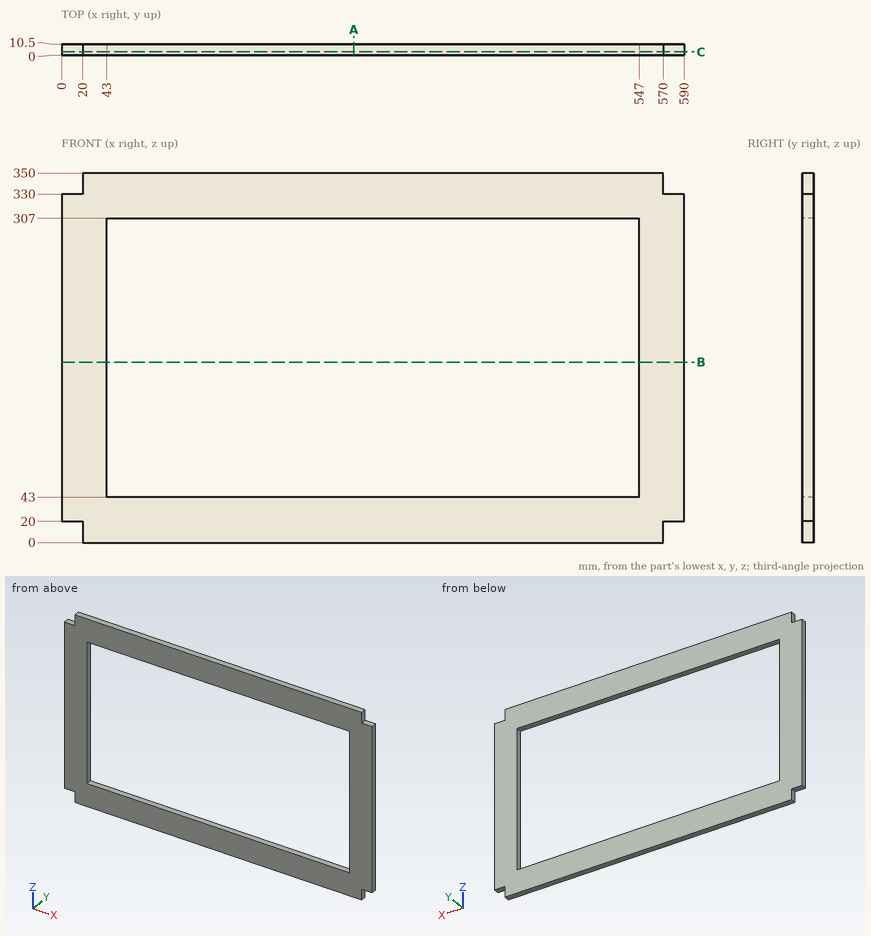
Can you work these out from the drawing? Everything is in mm from the part's minimum corner. Give positions to 0.01 mm unless a question says otherwise; leave off trailing zeros. Loops run counter-clockwise (first coordinate to the right, second up) from the corner with the lowest first, then second, coordinate; pieces in that order, holes last. Notation, with made-up numbers: (32.5, 36) -> (66.5, 36) arc R21 ccw to (66.5, 69) -> close; hole circle Ø10 at (12, 36). An arc over 180 degrees is marked (long way). Write item = value, one per line.
1) I need wall thicknesses on L1, parallel to X at y = 8, z = 279.5; L2, parallel to Z at x = 325.5, y = 8.75. Which ranges of each line are inside material? Lowest first, please. Write a range as from..to.
Check result:
L1 = 0..43, 547..590
L2 = 0..43, 307..350
2) Suppose I cut it at B-B on z = 171. Write out the boundary of the cut face in (x, y), then the cut area to 3 significant figures.
Check result:
outline = (0, 0) -> (43, 0) -> (43, 10.5) -> (0, 10.5) -> close; (547, 0) -> (590, 0) -> (590, 10.5) -> (547, 10.5) -> close
area = 903 mm2
3) Will these pins go through, and if not, where does the flat tip stop? pin 1 (5 mm diameter, centred on x = 579.5, y = 4, fed in from -Z); pin 2 (6 mm diameter, centred on x = 377.5, z = 302, fed in from -Y); pin 3 (3 mm diameter, centred on y = 5, z = 6.5, fed in from -X).
Check result:
pin_1 = 20
pin_2 = through
pin_3 = 20
4) Suppose I cut it at A-A on x = 277. Write out the boundary of the cut face in (y, z).
Check result:
outline = (0, 0) -> (10.5, 0) -> (10.5, 43) -> (0, 43) -> close; (0, 307) -> (10.5, 307) -> (10.5, 350) -> (0, 350) -> close
5) Suppose I cut it at C-C on y = 3. Write out the boundary of the cut face in (x, z), then the cut area to 3 significant figures.
Check result:
outline = (0, 20) -> (20, 20) -> (20, 0) -> (570, 0) -> (570, 20) -> (590, 20) -> (590, 330) -> (570, 330) -> (570, 350) -> (20, 350) -> (20, 330) -> (0, 330) -> close; hole (43, 43) -> (547, 43) -> (547, 307) -> (43, 307) -> close
area = 71,800 mm2
